Here's how the part is built. I have some questions about the finished solid (model axes, mm). Face numbers are marked on the shaded views. A direction names the side the tool comes from. Give positions to 0.01 mm unless a question says otherwise; leave off trailing zeros. Write each loop counter-clockwise with the first axis right and the second up, starting at its lowest first coordinate (ties: lowest second). Pieces come first, ordered by that corner, then holes. Notation, with made-up numbers: (72, -35.75) -> (108, -35.75) arc R15 ccw to (108, -23.75) -> close; hole circle Ø4 at (88, -26.5). An arc over 180 degrees is marked (long way). Use CSV: the item, a comma, the result in double quotes. Start each with the question number.
(1) If we mould it in two halves opening along Y, with no side actions, what happens to the marked faces 1, 2 and 3? For each: pulls with the +Y half, pulls with the -Y half, needs draft (parallel to the pull), parting line crosses it, or undercut.
(2) For pin 1 Ø1 at (x, y) = (-28.5, 27) entering from +Z, with a flat end and sliding along its axis, tell me the tip position at first contact or that it passes through.
(3) Suppose I cut it at D-D on x = 54.75. List the corners of the cut face in (y, z) for me, plus the area to 3 significant figures.
(4) Suppose I cut it at A-A on z = 23. List the corners of the cut face in (x, y) for me, plus the area to 3 significant figures.
(5) Suppose I cut it at B-B on z = 50. List the corners of the cut face in (x, y) for me.
(6) Suppose I cut it at C-C on x = -21. List the corners of the cut face in (y, z) for me, plus the area to 3 significant figures.
(7) Which directions (+Z, -Z, +X, -X, +Y, -Y) give clear straight access to the entire face, cutting with the end or side of a thin tool? Please do the marked faces 4 and 5.
(8) I need wall thicknesses on L1, parallel to X at y = -28, z = 91.5; L2, parallel to X at y = 1, z = 63; L3, parallel to Y at x = 8, z = 37. Which ranges of each line are inside material? Lowest first, please. Write a range as [from, to].
from build123d import *

# Parameters (mm, degrees)
F0_W      = 140.5
F0_H      = 90
F1_DEPTH  = 112
F2_T      = -5
F4_DEPTH  = 147.9
F6_DEPTH  = 83.1
F7_W      = 12
F7_H      = 12
F8_DEPTH  = 25
F9_W      = 130.5
F9_H      = 80
F10_DEPTH = 15
F11_W     = 90
F11_H     = 15
F12_DEPTH = 174.4
F14_DEPTH = 25
F15_W     = 13
F15_H     = 13
F16_DEPTH = 10
F18_DEPTH = 10
F20_DEPTH = 61.2


with BuildPart() as f1:
    # F0 (on Top) → F1 (new body)
    with BuildSketch(Plane.XY):
        Rectangle(F0_W, F0_H)
    extrude(amount=F1_DEPTH)

    # F2
    f2_openings = [f1.faces().sort_by_distance(p)[0] for p in [
        (0, 0, 112),
    ]]
    offset(amount=F2_T, openings=f2_openings)

    # F3 (on face) → F4 (cut)
    with BuildSketch(Plane(origin=(-70.25, 0, 0), x_dir=(0, -1, 0), z_dir=(-1, 0, 0))):
        with BuildLine():
            Line((-40.522967, 107), (-40, 107))
            Line((-40, 107), (40, 107))
            Line((40, 107), (40.522967, 107))
            ThreePointArc((40.522967, 107), (41.351034, 107.439371), (41.451444, 108.371391))
            Line((41.451444, 108.371391), (40.548556, 110.628609))
            ThreePointArc((40.548556, 110.628609), (40.648966, 111.560629), (41.477033, 112))
            Line((41.477033, 112), (-41.477033, 112))
            ThreePointArc((-41.477033, 112), (-40.648966, 111.560629), (-40.548556, 110.628609))
            Line((-40.548556, 110.628609), (-41.451444, 108.371391))
            ThreePointArc((-41.451444, 108.371391), (-41.351034, 107.439371), (-40.522967, 107))
        make_face()
    extrude(amount=-F4_DEPTH, mode=Mode.SUBTRACT)

    # F5 (on face) → F6 (join)
    with BuildSketch(Plane.XZ.offset(-40)):
        with BuildLine():
            ThreePointArc((65.25, 80.5), (54.75, 70), (44.25, 80.5))
            Line((44.25, 80.5), (44.25, 94.5))
            Line((44.25, 94.5), (41.75, 94.5))
            Line((41.75, 94.5), (41.75, 80.5))
            ThreePointArc((41.75, 80.5), (50.718871, 68.140793), (65.25, 72.835145))
            Line((65.25, 72.835145), (65.25, 80.5))
        make_face()
    extrude(amount=F6_DEPTH)

    # F7 (on face) → F8 (cut)
    with BuildSketch(Plane(origin=(0, -40, 0), x_dir=(-1, 0, 0), z_dir=(0, 1, 0))):
        with BuildLine():
            Line((-57.75, 112.14032), (-57.75, 80.5))
            ThreePointArc((-57.75, 80.5), (-54.75, 77.5), (-51.75, 80.5))
            Line((-51.75, 80.5), (-51.75, 112.14032))
            Line((-51.75, 112.14032), (-57.75, 112.14032))
        make_face()
        with Locations((-30.25, 89)):
            Rectangle(F7_W, F7_H)
        with Locations((-30.25, 72)):
            Rectangle(F7_W, F7_H)
    extrude(amount=-F8_DEPTH, mode=Mode.SUBTRACT)

    # F9 (on face) → F10 (join)
    with BuildSketch(Plane.XY.offset(5)):
        Rectangle(F9_W, F9_H)
    extrude(amount=F10_DEPTH)

    # F11 (on face) → F12 (cut)
    with BuildSketch(Plane(origin=(-70.25, 0, 0), x_dir=(0, -1, 0), z_dir=(-1, 0, 0))):
        with Locations((0, 7.5)):
            Rectangle(F11_W, F11_H)
        with BuildLine():
            ThreePointArc((15, 43.5), (21.5, 50), (15, 56.5))
            Line((15, 56.5), (-15, 56.5))
            ThreePointArc((-15, 56.5), (-21.5, 50), (-15, 43.5))
            Line((-15, 43.5), (15, 43.5))
        make_face()
    extrude(amount=-F12_DEPTH, mode=Mode.SUBTRACT)

    # F13 (on face) → F14 (cut)
    with BuildSketch(Plane(origin=(-70.25, 0, 0), x_dir=(0, -1, 0), z_dir=(-1, 0, 0))):
        with BuildLine():
            Line((-15, 78), (15, 78))
            ThreePointArc((15, 78), (21.5, 84.5), (15, 91))
            Line((15, 91), (-15, 91))
            ThreePointArc((-15, 91), (-21.5, 84.5), (-15, 78))
        make_face()
    extrude(amount=-F14_DEPTH, mode=Mode.SUBTRACT)

    # F15 (on face) → F16 (join)
    with BuildSketch(Plane.XY.offset(20)):
        with Locations((-53.75, 23)):
            Rectangle(F15_W, F15_H)
        with Locations((30.25, 23)):
            Rectangle(F15_W, F15_H)
        with Locations((30.25, -23)):
            Rectangle(F15_W, F15_H)
        with Locations((-53.75, -23)):
            Rectangle(F15_W, F15_H)
    extrude(amount=F16_DEPTH)

    # F17 (on face) → F18 (join)
    with BuildSketch(Plane.XY.offset(30)):
        Polygon((-47.25, 29.5), (-60.25, 29.5), (-60.25, 16.5), (-57.25, 16.5), (-57.25, 26.5), (-47.25, 26.5), align=None)
        Polygon((-60.25, -29.5), (-47.25, -29.5), (-47.25, -26.5), (-57.25, -26.5), (-57.25, -16.5), (-60.25, -16.5), align=None)
        Polygon((33.75, 26.5), (33.75, 16.5), (36.75, 16.5), (36.75, 29.5), (23.75, 29.5), (23.75, 26.5), align=None)
        Polygon((23.75, -26.5), (23.75, -29.5), (36.75, -29.5), (36.75, -16.5), (33.75, -16.5), (33.75, -26.5), align=None)
    extrude(amount=F18_DEPTH)

    # F19 (on Front) → F20 (cut)
    with BuildSketch(Plane.XZ):
        Polygon((-63.45, 90), (-63.45, 78), (-58.946795, 78), (-54.15, 78), (-54.15, 90), align=None)
    extrude(amount=-F20_DEPTH, mode=Mode.SUBTRACT)


solid = f1.part
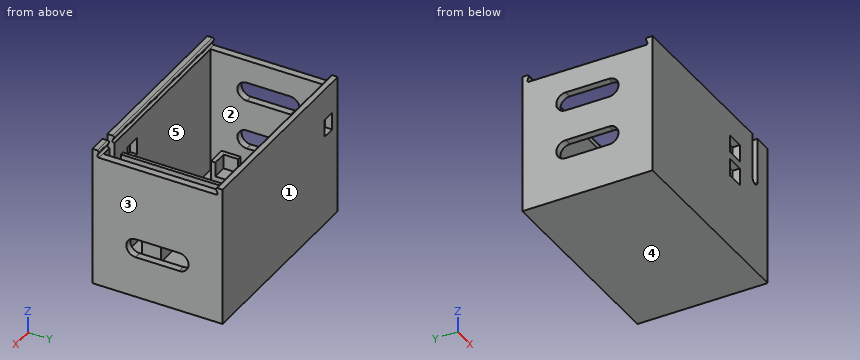
Geometry says:
1,face 1,"pulls with the +Y half"
1,face 2,"undercut"
1,face 3,"needs draft"
2,pin 1,"z = 20"
3,outline,"(-45, 15) -> (45, 15) -> (45, 112) -> (41.48, 112) arc R1 ccw to (40.55, 110.63) -> (41.45, 108.37) arc R1 cw to (40.52, 107) -> (40, 107) -> (40, 70) -> (-40, 70) -> (-40, 77.5) -> (-45, 77.5) -> close; hole (-40, 20) -> (40, 20) -> (40, 67.5) -> (-40, 67.5) -> close"
3,area,"1,390 mm²"
4,outline,"(-70.25, -45) -> (70.25, -45) -> (70.25, 45) -> (-70.25, 45) -> close; (-60.25, -29.5) -> (-47.25, -29.5) -> (-47.25, -16.5) -> (-60.25, -16.5) -> close; (-60.25, 16.5) -> (-47.25, 16.5) -> (-47.25, 29.5) -> (-60.25, 29.5) -> close; (23.75, -29.5) -> (36.75, -29.5) -> (36.75, -16.5) -> (23.75, -16.5) -> close; (23.75, 16.5) -> (36.75, 16.5) -> (36.75, 29.5) -> (23.75, 29.5) -> close; hole (-65.25, -40) -> (65.25, -40) -> (65.25, 40) -> (-65.25, 40) -> close"
4,area,"2,880 mm²"
5,outline,"(-70.25, -45) -> (70.25, -45) -> (70.25, -21.5) -> (65.25, -21.5) -> (65.25, -40) -> (-65.25, -40) -> (-65.25, -21.5) -> (-70.25, -21.5) -> close; (-70.25, 21.5) -> (-65.25, 21.5) -> (-65.25, 40) -> (65.25, 40) -> (65.25, 21.5) -> (70.25, 21.5) -> (70.25, 45) -> (-70.25, 45) -> close"
6,outline,"(-45, 15) -> (45, 15) -> (45, 112) -> (41.48, 112) arc R1 ccw to (40.55, 110.63) -> (41.45, 108.37) arc R1 cw to (40.52, 107) -> (40, 107) -> (40, 20) -> (-40, 20) -> (-40, 107) -> (-40.52, 107) arc R1 cw to (-41.45, 108.37) -> (-40.55, 110.63) arc R1 ccw to (-41.48, 112) -> (-45, 112) -> close"
6,area,"1,360 mm²"
7,face 4,"-Z, +X, -X, +Y, -Y"
7,face 5,"none"
8,L1,"[-70.25, -65.25], [41.75, 44.25], [65.25, 70.25]"
8,L2,"[-70.25, -65.25], [65.25, 70.25]"
8,L3,"[-45, -40], [40, 45]"
